from build123d import *

# Parameters (mm, degrees)
SKETCH_1_R          = 10
EXTRUDE_1_DEPTH     = 5
SKETCH_2_R          = 75
CUT_EXTRUDE_1_DEPTH = 167.952088936


with BuildPart() as part:
    # 草图1 → 凸台-拉伸1 (new body)
    with BuildSketch(Plane(origin=(0, 0, 0), x_dir=(1, 0, 0), z_dir=(0, 1, 0))):
        with BuildLine():
            Line((-100, 118), (100, 118))
            ThreePointArc((100, 118), (112.727922061, 112.727922061), (118, 100))
            Line((118, 100), (118, -100))
            ThreePointArc((118, -100), (112.727922061, -112.727922061), (100, -118))
            Line((100, -118), (-100, -118))
            ThreePointArc((-100, -118), (-112.727922061, -112.727922061), (-118, -100))
            Line((-118, -100), (-118, 100))
            ThreePointArc((-118, 100), (-112.727922061, 112.727922061), (-100, 118))
        make_face()
        with Locations(Location((100, 100, 0), (0, 0, 270))):
            Circle(SKETCH_1_R, mode=Mode.SUBTRACT)
        with Locations(Location((100, -100, 0), (0, 0, 270))):
            Circle(SKETCH_1_R, mode=Mode.SUBTRACT)
        with Locations(Location((-100, -100, 0), (0, 0, 270))):
            Circle(SKETCH_1_R, mode=Mode.SUBTRACT)
        with Locations(Location((-100, 100, 0), (0, 0, 270))):
            Circle(SKETCH_1_R, mode=Mode.SUBTRACT)
    extrude(amount=EXTRUDE_1_DEPTH)

    # 草图2 → 切除-拉伸1 (cut, through all)
    with BuildSketch(Plane.XZ):
        with Locations(Location((0, 0, 0), (0, 0, 270))):
            Circle(SKETCH_2_R)
    extrude(amount=-CUT_EXTRUDE_1_DEPTH, mode=Mode.SUBTRACT)


solid = part.part
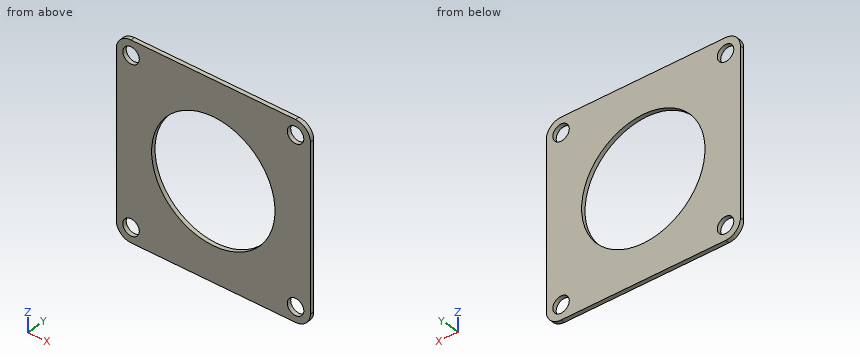
Model file for the job. Use its own axes, mm. Coordinates: 2 decimals unless noted, no trailing zeros. Order: outer loops, then holes, each group sorted by start corner. A loop starts at its lowest first (then second) coordinate and runs counter-clockwise, first axis right, second up. Notation, with made-up numbers: M 13,8 L 71,8 A20 cw 71,29 Z; hole C -37,-17.5 d6. An arc over 180 degrees is marked long. Return JSON: item names as keys, results as strings.
1. Saw through at C-C (z = 48). Give the cut face in (x, y), and give its area (3 significant figures).
Ans:
{"outline": "M -118,0 L -57.63,0 L -57.63,5 L -118,5 Z; M 57.63,0 L 118,0 L 118,5 L 57.63,5 Z", "area": "604 mm^2"}
2. Saw through at A-A (y = 1.55). Give the cut face in (x, z), and give its area (3 significant figures).
Ans:
{"outline": "M -118,-100 A18 ccw -100,-118 L 100,-118 A18 ccw 118,-100 L 118,100 A18 ccw 100,118 L -100,118 A18 ccw -118,100 Z; hole C -100,-100 d20; hole C -100,100 d20; hole C 0,0 d150; hole C 100,-100 d20; hole C 100,100 d20", "area": "36,500 mm^2"}
3. Saw through at B-B (x = 0). Give the cut face in (y, z), and give its area (3 significant figures).
Ans:
{"outline": "M 0,-118 L 5,-118 L 5,-75 L 0,-75 Z; M 0,75 L 5,75 L 5,118 L 0,118 Z", "area": "430 mm^2"}
4. Drill centre lines: probe 1 along X at (y, z) = (2.8, 100); probe 2 along Z at (x, y) = (104.5, 2.15); probe 3 along X at (y, z) = (1.8, 10). Where is each one in solid material? Low to high.
Ans:
{"probe 1": "-118 to -110, -90 to 90, 110 to 118", "probe 2": "-117.43 to -108.93, -91.07 to 91.07, 108.93 to 117.43", "probe 3": "-118 to -74.33, 74.33 to 118"}
